The listing builds one solid part. Answer for the finished solid, in the listing's coordinates (mm). A direction names the side the tool comes from. Give positions to 0.01 mm unless a question says otherwise; leave off trailing zeros. Loops run counter-clockwise (first coordinate to the right, second up) from the corner with the lowest first, then second, coordinate; pieces in that order, holes last.
Item 1: The mould has two halves that part along X. Classify faces 1 (the face through (187, 10, 0)), 2 (the face through (380, 10, -345)), 3 (the face through (190, 10, -60)): pulls with the +X half, pulls with the -X half, needs draft (parallel to the pull), parting line crosses it, or undercut.
Item 2: A tool of negligible diameter and unlimited length cuts with its end or side. For faces 4 (the face through (187, 20, -355)), 5 (the face through (190, 10, -80)), from which of +Z, -Z, +X, -X, +Y, -Y can it reach the whole face along a straight path? Write none if from no direction.
Item 3: Section A-A, the plane x = 179 is taken. Give the vertices of the cut face in (y, z), and give its area (3 significant figures).
Item 4: Consider line 1 along Z through (x, y) = (179, 17.25). Determine where the line is inside the solid, lowest interval first.
from build123d import *

# Parameters (mm, degrees)
EXTRUDE_1_DEPTH     = 20
SKETCH_2_W          = 336
SKETCH_2_H          = 230
CUT_EXTRUDE_1_DEPTH = 20
CUT_EXTRUDE_2_DEPTH = 20


with BuildPart() as part:
    # 草图1 → 凸台-拉伸1 (new body)
    with BuildSketch(Plane(origin=(0, 0, 0), x_dir=(1, 0, 0), z_dir=(0, 1, 0))):
        Polygon((0, 0), (380, 0), (716, 0), (716, 230), (380, 230), (380, 700), (0, 700), align=None)
    extrude(amount=EXTRUDE_1_DEPTH)

    # 草图2 → 切除-拉伸1 (cut)
    with BuildSketch(Plane(origin=(0, 20, 0), x_dir=(1, 0, 0), z_dir=(0, 1, 0))):
        with Locations((548, 115)):
            Rectangle(SKETCH_2_W, SKETCH_2_H)
    extrude(amount=-CUT_EXTRUDE_1_DEPTH, mode=Mode.SUBTRACT)

    # 草图3 → 切除-拉伸2 (cut)
    with BuildSketch(Plane(origin=(0, 20, 0), x_dir=(1, 0, 0), z_dir=(0, 1, 0))):
        with BuildLine():
            Line((171, 80), (209, 80))
            ThreePointArc((209, 80), (213.242640687, 78.242640687), (215, 74))
            Line((215, 74), (215, 66))
            ThreePointArc((215, 66), (213.242640687, 61.757359313), (209, 60))
            Line((209, 60), (171, 60))
            ThreePointArc((171, 60), (166.757359313, 61.757359313), (165, 66))
            Line((165, 66), (165, 74))
            ThreePointArc((165, 74), (166.757359313, 78.242640687), (171, 80))
        make_face()
    extrude(amount=-CUT_EXTRUDE_2_DEPTH, mode=Mode.SUBTRACT)


solid = part.part
Worked answers:
1. face 1: needs draft
1. face 2: pulls with the +X half
1. face 3: undercut
2. face 4: +Z, -Z, +X, -X, +Y
2. face 5: +Y, -Y
3. outline: (0, -700) - (20, -700) - (20, -80) - (0, -80) - close; (0, -60) - (20, -60) - (20, 0) - (0, 0) - close
3. area: 13,600 mm2
4. line 1: z = -700 to -80, -60 to 0
